Autodesk Inventor part; units mm, degrees
ref_plane "YZ Plane" through (0, 0, 0) normal (1, 0, 0) x (0, 1, 0)
ref_plane "XZ Plane" through (0, 0, 0) normal (0, 1, 0) x (-1, 0, 0)
ref_plane "XY Plane" through (0, 0, 0) normal (0, 0, 1) x (1, 0, 0)
sketch "Sketch3" plane through (0, 0, 0) normal (0, 0, 1) x (1, 0, 0)
  circle A0 centre (0, 0) radius 2
  line L0 (1.0225, 0.5903) -> (1.0225, -0.5903)
  line L1 (1.0225, -0.5903) -> (0, -1.1807)
  line L2 (0, -1.1807) -> (-1.0225, -0.5903)
  line L3 (-1.0225, -0.5903) -> (-1.0225, 0.5903)
  line L4 (-1.0225, 0.5903) -> (0, 1.1807)
  line L5 (0, 1.1807) -> (1.0225, 0.5903)
  line L6 (0, 0) -> (0, 1.1807) construction
  dimension "HexWidth" = 2.045
sketch "Sketch2" plane through (0, 0, 0) normal (0, 0, 1) x (1, 0, 0)
  circle A0 centre (0, 0) radius 2
  dimension "Diam" = 4
extrude "Extrusion2" add sketch "Sketch2" against normal blind 20
thread "Thread1"
extrude "Extrusion3" cut sketch "Sketch3" against normal blind 2.5 contours L0 L1 L2 L3 L4 L5
chamfer "Chamfer2" distance 0.75 angle 45 1 edges at (-2, 0, -20)
chamfer "Chamfer3" distance 0.1875 angle 45 1 edges at (-2, 0, 0)
sketch "Sketch4" plane through (0, 0, -20) normal (0, 0, -1) x (-1, 0, 0)
  circle A0 centre (0, 0) radius 1.8125
hole "Cup_Point_Hole1" at (0, 0, -20) direction (0, 0, 1) diameter 2.4999 depth 0.001 tip angle 118
equation "\"d8\" = -0.5 * CupPointDiam + 0.5 * Diam"
equation "\"d11\" = 0.25 * d8"
equation "\"CupPointDiam\" = 2.5"
properties part number "SCREW,SET,CUP POINT,P, 8.8, M4X0.7X20MM" material "Steel, MS"
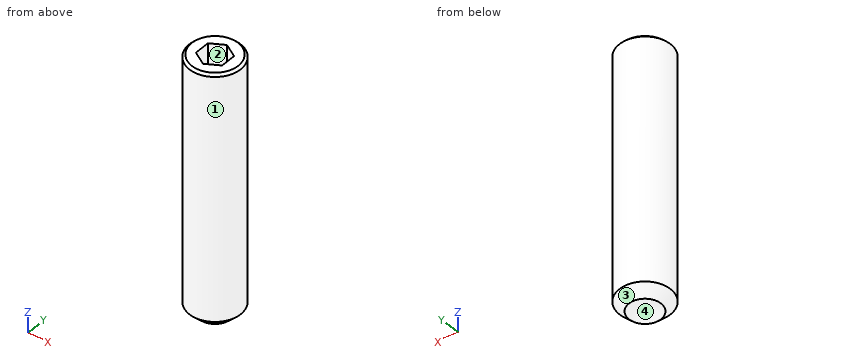
For this review, take the finished solid that the model builds, in its own axes (mm). Face numbers are marked on the shaded views. A direction names the side the tool comes from. Round coordinates to 2 decimals unless told otherwise and drop trailing zeros. Loops run counter-clockwise (first coordinate to the right, second up) from the corner with the lowest first, then second, coordinate; pieces in that order, holes last. Notation, with made-up numbers: (21.25, -12) - (36.25, -12) arc R26 cw to (36.25, 27) - close; hole circle Ø7 at (53.25, 18). An arc over 180 degrees is marked (long way). One line per question, with ' | ' between items.
Q1. For line 1 along Y through (x, z) = (0.7, -1.25); line 2 along Y through (x, z) = (0.75, -0.75); line 3 along X through (y, z) = (1.75, -17), list the stretches that pass through material, from the lowest coordinate up. Write a range as [from, to].
Taken from the geometry:
line 1: y = [-1.87, -0.78], [0.78, 1.87] | line 2: y = [-1.85, -0.75], [0.75, 1.85] | line 3: x = [-0.97, 0.97]
Q2. For pin 1 (2 mm diameter, centred on x = 0, y = 0, fed in from -Z), flat-tipped, find the tip position at first contact; note if it passes through.
Taken from the geometry:
pin 1: stops at z = -19.85
Q3. The part is to be moulded in two halves that separate along X. For the marked faces 3 and 4, say which applies: released by +X, released by -X, zero draft, split by the parting line, or undercut.
Taken from the geometry:
face 3: split by the parting line | face 4: undercut
Q4. Tool access review of the marked faces 1 and 2: name each direction out of +Z, -Z, +X, -X, +Y, -Y from which nothing blocks a thin tool from reaching the whole face with its end or side.
Taken from the geometry:
face 1: +Z, -Z | face 2: +Z
Q5. Take a section at A-A (z = -14.25). Give the boundary of the cut face in (x, y).
Taken from the geometry:
outline: circle Ø4 at (0, 0)
